The model under review builds one solid part; all positions refer to its coordinate system, in mm. A direction names the side the tool comes from. Coordinates: 2 decimals unless noted, no trailing zeros. Order: outer loops, then holes, each group sorted by start corner. A loop starts at its lowest first (then second) coordinate and runs counter-clockwise, first axis right, second up. Notation, with made-up numbers: M 66,-5 L 95,-5 A9 ccw 95,-1 Z; hole C 16.25,78.25 d10. An arc over 180 degrees is marked long. One line per item, written item: value.
Autodesk Inventor part; units mm, degrees
ref_plane "YZ Plane" through (0, 0, 0) normal (1, 0, 0) x (0, 1, 0)
ref_plane "XZ Plane" through (0, 0, 0) normal (0, 1, 0) x (-1, 0, 0)
ref_plane "XY Plane" through (0, 0, 0) normal (0, 0, 1) x (1, 0, 0)
sketch "Sketch1" plane through (0, 0, 0) normal (0, 0, 1) x (1, 0, 0)
  line L0 (-6.35, -6.35) -> (6.35, -6.35)
  line L1 (6.35, -6.35) -> (6.35, 6.35)
  line L2 (6.35, 6.35) -> (-6.35, 6.35)
  line L3 (-6.35, 6.35) -> (-6.35, -6.35)
  line L4 (-6.35, -6.35) -> (6.35, 6.35) construction
  line L5 (6.35, -6.35) -> (-6.35, 6.35) construction
  line L6 (-4.7625, -4.7625) -> (4.7625, -4.7625)
  line L7 (4.7625, -4.7625) -> (4.7625, 4.7625)
  line L8 (4.7625, 4.7625) -> (-4.7625, 4.7625)
  line L9 (-4.7625, 4.7625) -> (-4.7625, -4.7625)
  line L10 (-4.7625, -4.7625) -> (4.7625, 4.7625) construction
  line L11 (4.7625, -4.7625) -> (-4.7625, 4.7625) construction
  point P0 (0, 0)
  point P1 (0, 0)
  dimension "d0" = 12.7
  dimension "d1" = 12.7
  dimension "d2" = 9.525
  dimension "d3" = 9.525
extrude "Extrusion1" add sketch "Sketch1" along normal blind 203.2
sketch "Sketch2" plane through (6.35, -6.35, 0) normal (1, 0, 0) x (0, 0, -1)
  line L0 (0, 0) -> (-203.2, 0)
  circle A0 centre (-13.3193, 6.35) radius 2.413
  circle A1 centre (-91.9323, 6.35) radius 2.413
  line L1 (-89.5193, 6.35) -> (-13.3193, 6.35)
  point P0 (0, 6.35)
  dimension "d7" = 4.826
  dimension "d6" = 4.826
  dimension "d8" = 76.2
extrude "Extrusion2" cut sketch "Sketch2" against normal blind 203.2
properties part number "custom box alluminum 8in"
(1) We need section A-A, the plane y = 0. State the section outline as (x, z) points.
Geometry results:
outline: M -6.35,0 L -4.76,0 L -4.76,10.91 L -6.35,10.91 Z; M -6.35,15.73 L -4.76,15.73 L -4.76,89.52 L -6.35,89.52 Z; M -6.35,94.35 L -4.76,94.35 L -4.76,203.2 L -6.35,203.2 Z; M 4.76,0 L 6.35,0 L 6.35,10.91 L 4.76,10.91 Z; M 4.76,15.73 L 6.35,15.73 L 6.35,89.52 L 4.76,89.52 Z; M 4.76,94.35 L 6.35,94.35 L 6.35,203.2 L 4.76,203.2 Z
(2) We need section B-B, the plane x = -1. State the section outline as (y, z) points, plus the area to 3 significant figures.
Geometry results:
outline: M -6.35,0 L -4.76,0 L -4.76,203.2 L -6.35,203.2 Z; M 4.76,0 L 6.35,0 L 6.35,203.2 L 4.76,203.2 Z
area: 645 mm2
(3) Tool access review of faces 1 (the flat face through (6, 0, 203.2)), 2 (the flat face through (4.762, 0, 100)): name each direction out of +Z, -Z, +X, -X, +Y, -Y from which nothing blocks a thin tool from reaching the whole face with its end or side.
Geometry results:
face 1: +Z, +X, -X, +Y, -Y
face 2: +Z, -Z
(4) For L1, parallel to Y at x = -3.25, z = 145, list the stretches that pass through material, from the lowest coordinate up.
Geometry results:
L1: y = -6.35 to -4.76, 4.76 to 6.35
(5) We need section C-C, the plane z = 134. State the section outline as (x, y) points, plus the area to 3 significant figures.
Geometry results:
outline: M -6.35,-6.35 L 6.35,-6.35 L 6.35,6.35 L -6.35,6.35 Z; hole M -4.76,-4.76 L 4.76,-4.76 L 4.76,4.76 L -4.76,4.76 Z
area: 70.6 mm2
(6) Mouldability with a two-part tool opening along X and no side actions: class faces 3 (the flat face through (0, -4.762, 100)), 4 (the flat face through (-6.35, 0, 100)), 5 (the flat face through (-4.762, 0, 100)), 6 (the flat face through (6.35, 0, 100)) as +X half, -X half, draft (parallel to the pull), parting line (faces both ways), or undercut.
Geometry results:
face 3: undercut
face 4: -X half
face 5: undercut
face 6: +X half
(7) Insertion check: pin 1 Ø1 at (x, y) = (2, 4) entering from +Z. The pin has a flat end and moves straight along its axis. Give the tip position at first contact, or say it passes through.
Geometry results:
pin 1: passes through
